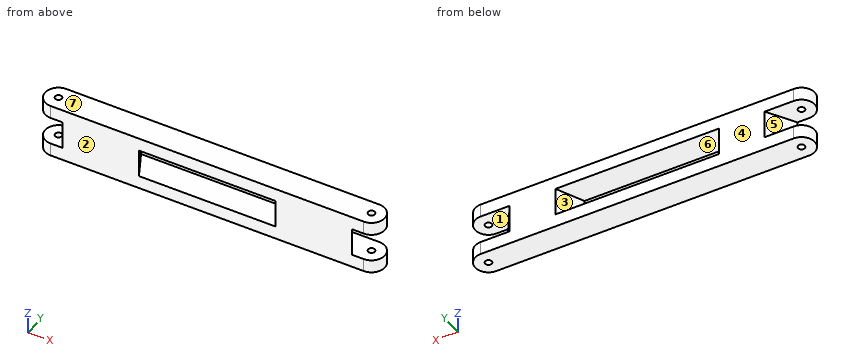
from build123d import *

# Parameters (mm, degrees)
F0_R     = 0.75
F1_DEPTH = 3
F3_DEPTH = 3.2


with BuildPart() as f1:
    # F0 (on Top) → F1 (new body)
    with BuildSketch(Plane.XY):
        with BuildLine():
            ThreePointArc((35, -3), (38, 0), (35, 3))
            Line((35, 3), (-35, 3))
            ThreePointArc((-35, 3), (-38, 0), (-35, -3))
            Line((-35, -3), (35, -3))
        make_face()
        with Locations((-35, 0)):
            Circle(F0_R, mode=Mode.SUBTRACT)
        with Locations((35, 0)):
            Circle(F0_R, mode=Mode.SUBTRACT)
    extrude(amount=F1_DEPTH)

    # F2 (on face) → F3 (join)
    with BuildSketch(Plane.XY.offset(3)):
        Polygon((-28.517587, 3), (-32.340631, -3), (-15.273468, -3), (-18.277289, 3), align=None)
        Polygon((18.277289, 3), (15.273468, -3), (32.340631, -3), (28.517587, 3), align=None)
    extrude(amount=F3_DEPTH)

    # F4: F1 across face


with BuildPart() as f1_1:
    add(f1.part)
    add(f1.part.mirror(Plane(origin=(23.619311, -0.25, 6.2), x_dir=(1, 0, 0), z_dir=(0, 0, 1))))


solid = f1_1.part
Check sheet for the modelled part. Datum: model origin and axes. Units: mm. Face numbers are marked on the shaded views. A direction names the side the tool comes from. Round coordinates to 2 decimals unless told otherwise and drop trailing zeros. Loops run counter-clockwise (first coordinate to the right, second up) from the corner with the lowest first, then second, coordinate; pieces in that order, holes last. Notation, with made-up numbers: (71.5, 31) -> (103.5, 31) arc R16 cw to (103.5, 35) -> close; hole circle Ø10 at (46, -10.5). An arc over 180 degrees is marked (long way). Put each result on its own line as item: value. Start each with the question number.
1. Access from +Z, -Z, +X, -X, +Y, -Y to the whole of each face (thin tool, end or side, straight path). Record for the marked faces 1, 2, 3 and 4.
2. Section check B-B (z = 11.5). Enter the section's corners in (x, y).
3. Draft check along X on the marked faces 5, 6 and 7. Enter one of: +X half, -X half, draft (parallel to the pull), parting line (faces both ways), or undercut.
4. Section check D-D (x = -29.5). Enter the section's corners in (y, z).
5. Scan lines: probe 1 along X at (y, z) = (-0.05, 2.75); probe 2 along Z at (x, y) = (11.5, -1.1); probe 3 along Y at (x, z) = (-35, 2.1). Record each from-to range of solid material in increasing order.
6. Section check C-C (y = 0). Give the number of separate pieces and of enclosed holes in the cut face, plus the area to 3 significant figures.
7. Section check A-A (x = 8.5). Enter the section's corners in (y, z).
Findings:
1. face 1: +X, +Y
1. face 2: +Z, -Z, +X, -X, -Y
1. face 3: +Y
1. face 4: +Z, -Z, +X, -X, +Y
2. outline: (-35, -3) -> (35, -3) arc R3 ccw to (35, 3) -> (-35, 3) arc R3 ccw to start; hole circle Ø1.5 at (-35, 0); hole circle Ø1.5 at (35, 0)
3. face 5: -X half
3. face 6: undercut
3. face 7: draft
4. outline: (-3, 0) -> (3, 0) -> (3, 3) -> (1.46, 3) -> (1.46, 9.4) -> (3, 9.4) -> (3, 12.4) -> (-3, 12.4) -> close
5. probe 1: x = -38 to -35.75, -34.25 to 34.25, 35.75 to 38
5. probe 2: z = 0 to 3, 9.4 to 12.4
5. probe 3: y = -3 to -0.75, 0.75 to 3
6. separate pieces: 5
6. enclosed holes: 1
6. area: 613 mm^2
7. outline: (-3, 0) -> (3, 0) -> (3, 3) -> (-3, 3) -> close; (-3, 9.4) -> (3, 9.4) -> (3, 12.4) -> (-3, 12.4) -> close
